from build123d import *

# Parameters (mm, degrees)
F2_R     = 3.175
F3_DEPTH = 19.05


with BuildPart() as f1:
    # F0 (on Right) → F1 (revolve)
    with BuildSketch(Plane.YZ):
        Polygon((-11.863786, 3.175), (-11.863786, 0), (13.536214, 0), (13.536214, 3.175), (10.996214, 3.175), (10.996214, 11.1125), (-9.323786, 11.1125), (-9.323786, 3.175), align=None)
    revolve(axis=Axis((0, 2.995029, 0), (0, 1, 0)))

    # F2 (on Right) → F3 (cut, symmetric)
    with BuildSketch(Plane.YZ):
        with Locations((0.725993, 0)):
            Circle(F2_R)
    extrude(amount=F3_DEPTH, both=True, mode=Mode.SUBTRACT)


solid = f1.part
Can you work these out from the model? Positions are in its coordinate system, mm. A direction names the side the tool comes from. Coordinates: 2 decimals unless noted, no trailing zeros. Write each loop counter-clockwise with the first axis right and the second up, starting at its lowest first coordinate (ties: lowest second). Pieces come first, ordered by that corner, then holes. Notation, with made-up numbers: (-36, 61.5) -> (16, 61.5) arc R10 ccw to (16, 66.5) -> close; hole circle Ø8 at (67, -3.75). An arc over 180 degrees is marked (long way). Write each question's results on one line, items separated by ' | '. Start each with the question number.
Item 1: Thinking about a two-plate mould opening in Z: for faces 4 (the cylindrical face through (-9.859, 0.694, 5.128)), 5 (the flat face through (-2, 10.996, 3)), 6 (the cylindrical face through (0.156, -1.794, -1.932)), which applies, released by +Z, released by -Z, zero draft, split by the parting line, or undercut?
Item 2: On a 3-axis mill with a long thin cutter (end or side, diameter ignored), from which of +Z, -Z, +X, -X, +Y, -Y can I reach the whole of each face in a straight line? I mean faces 1 (the flat face through (0, 13.536, 0)), 2 (the cylindrical face through (-3.1, -10.61, -0.69)), 3 (the cylindrical face through (-3.1, 12.25, -0.69)). Say none if no direction works.
Item 3: If we section it at D-D, the plane x = 2.5: Write out the boundary of the cut face in (y, z) (3 decimals).
Item 4: If we section it at A-A, the plane z = 0: Write out the boundary of the cut face in (x, y) (1 decimal).
Item 5: I'm going to push flat-ended pins straight in: P1, Ø5, axis at x = -4.5, y = -2, coming from the -Z side; P2, Ø3, axis at y = -5, z = 7, coming from the -X side; P3, Ø4, axis at x = 4, y = 1, coming from the +Z side. Where does each tip first touch, or does it pass through?
Item 6: If we section it at C-C, the plane y = 2: Write out the boundary of the cut face in (x, z) (1 decimal), and give its area (3 significant figures).
Item 7: Please list where these lines run through material, in increasing order: probe 1 along Y at (x, z) = (-2, 5.75); probe 2 along Y at (x, z) = (3, 0); probe 3 along Y at (x, z) = (-1, -2.75).
Answer block:
1) face 4: split by the parting line | face 5: zero draft | face 6: undercut
2) face 1: +Z, -Z, +X, -X, +Y | face 2: -Y | face 3: +Y
3) outline: (-11.864, -1.957) -> (-9.324, -1.957) -> (-9.324, -10.828) -> (10.996, -10.828) -> (10.996, -1.957) -> (13.536, -1.957) -> (13.536, 1.957) -> (10.996, 1.957) -> (10.996, 10.828) -> (-9.324, 10.828) -> (-9.324, 1.957) -> (-11.864, 1.957) -> close; hole circle Ø6.35 at (0.726, 0)
4) outline: (-11.1, -9.3) -> (-3.2, -9.3) -> (-3.2, -11.9) -> (3.2, -11.9) -> (3.2, -9.3) -> (11.1, -9.3) -> (11.1, -2.4) -> (-11.1, -2.4) -> close; (-11.1, 3.9) -> (11.1, 3.9) -> (11.1, 11) -> (3.2, 11) -> (3.2, 13.5) -> (-3.2, 13.5) -> (-3.2, 11) -> (-11.1, 11) -> close
5) P1: z = -10.93 | P2: x = -9.66 | P3: z = 10.93
6) outline: (-10.7, -2.9) arc R11.1 ccw to (10.7, -2.9) -> close; (-10.7, 2.9) -> (10.7, 2.9) arc R11.1 ccw to start | area: 260 mm²
7) probe 1: -9.32 to 11 | probe 2: -11.86 to -2.45, 3.9 to 13.54 | probe 3: -11.86 to -0.86, 2.31 to 13.54
